Can you work these out from the model? Positions are in its coordinate system, mm. A direction names the side the tool comes from. Round coordinates to 2 decimals unless told otherwise and drop trailing zeros. Loops run counter-clockwise (first coordinate to the right, second up) from the corner with the lowest first, then second, coordinate; pieces in that order, holes last. Notation, with made-up numbers: M 16,42.25 L 43,42.25 A27 cw 43,79.25 Z; hole C 16.5,-22.75 d7. An arc over 180 degrees is marked long. Return JSON: item names as keys, results as strings.
```python
from build123d import *

# Parameters (mm, degrees)
SKETCH1_W           = 40
SKETCH1_H           = 40
BOSS_EXTRUDE1_DEPTH = 3.5
SKETCH2_R           = 1.5
BOSS_EXTRUDE2_DEPTH = 14


with BuildPart() as part:
    # Sketch1 → Boss-Extrude1 (new body)
    with BuildSketch(Plane(origin=(0, 0, 0), x_dir=(1, 0, 0), z_dir=(0, 1, 0))):
        Rectangle(SKETCH1_W, SKETCH1_H)
    extrude(amount=BOSS_EXTRUDE1_DEPTH)

    # Sketch2 → Boss-Extrude2 (add)
    with BuildSketch(Plane.XY.offset(20)):
        with Locations((18.25, 1.75)):
            Circle(SKETCH2_R)
        with Locations(Location((-18.25, 1.75, 0), (0, 0, 180))):
            Circle(SKETCH2_R)
    extrude(amount=BOSS_EXTRUDE2_DEPTH)


solid = part.part
```
Q1. Suppose I cut it at A-A, the plane y = 1.75. Please give me the cut outline in (x, z).
Results:
{"outline": "M -20,-20 L 20,-20 L 20,20 L 19.75,20 L 19.75,34 L 16.75,34 L 16.75,20 L -16.75,20 L -16.75,34 L -19.75,34 L -19.75,20 L -20,20 Z"}
Q2. Suppose I cut it at C-C, the plane z = 23. Please give me the cut outline in (x, y).
Results:
{"outline": "C -18.25,1.75 d3; C 18.25,1.75 d3"}
Q3. Thinking about a two-plate mould opening in X: for faces 1 (the flat face through (0, 0, 0)), 2 (the cylindrical face through (-16.75, 1.68, 26.9)), 3 (the flat face through (20, 2, 0)), 4 (the flat face through (0, 2, 20)), which applies, pulls with the +X half, pulls with the -X half, needs draft (parallel to the pull), parting line crosses it, or undercut?
Results:
{"face 1": "needs draft", "face 2": "undercut", "face 3": "pulls with the +X half", "face 4": "undercut"}
Q4. If I drill on line 1 along X through (y, z) = (1.8, 24); line 2 along Z through (x, y) = (-12, 1.05); line 3 along X through (y, z) = (2.7, 26), over which ranges is the centre line in solid material (lowest first)?
Results:
{"line 1": "x = -19.75 to -16.75, 16.75 to 19.75", "line 2": "z = -20 to 20", "line 3": "x = -19.41 to -17.09, 17.09 to 19.41"}
Q5. On a 3-axis mill with a long thin cutter (end or side, diameter ignored), from which of +Z, -Z, +X, -X, +Y, -Y can I reach the whole of each face in a straight line? I mean faces 5 (the cylindrical face through (16.75, 1.82, 26.9)), 6 (the flat face through (-18, 2, 34)). Say none if no direction works.
Results:
{"face 5": "+Z", "face 6": "+Z, +X, -X, +Y, -Y"}
Q6. Suppose I cut it at D-D, the plane x = 14. Please give me the cut outline in (y, z), plus the area to 3 significant figures.
Results:
{"outline": "M 0,-20 L 3.5,-20 L 3.5,20 L 0,20 Z", "area": "140 mm2"}
Q7. Suppose I cut it at B-B, the plane x = 18.25. Please give me the cut outline in (y, z).
Results:
{"outline": "M 0,-20 L 3.5,-20 L 3.5,20 L 3.25,20 L 3.25,34 L 0.25,34 L 0.25,20 L 0,20 Z"}
